from build123d import *

# Parameters (mm, degrees)
EXTRUDE_1_DEPTH = 5


with BuildPart() as part:
    # 草图1 → 凸台-拉伸1 (new body)
    with BuildSketch(Plane(origin=(0, 0, 0), x_dir=(0, 0, -1), z_dir=(1, 0, 0))):
        Polygon((0, 0), (-250, 0), (-250, 20), (-245, 20), (-245, 50), (-250, 50), (-250, 70), (0, 70), (0, 50), (-5, 50), (-5, 20), (0, 20), align=None)
        with BuildLine():
            Line((-228.2219096, 66), (-20.2219096, 66))
            ThreePointArc((-20.2219096, 66), (-19.514802819, 65.707106781), (-19.2219096, 65))
            Line((-19.2219096, 65), (-19.2219096, 64))
            ThreePointArc((-19.2219096, 64), (-19.514802819, 63.292893219), (-20.2219096, 63))
            Line((-20.2219096, 63), (-228.2219096, 63))
            ThreePointArc((-228.2219096, 63), (-228.929016382, 63.292893219), (-229.2219096, 64))
            Line((-229.2219096, 64), (-229.2219096, 65))
            ThreePointArc((-229.2219096, 65), (-228.929016382, 65.707106781), (-228.2219096, 66))
        make_face(mode=Mode.SUBTRACT)
        with BuildLine():
            Line((-228.2219096, 4), (-20.2219096, 4))
            ThreePointArc((-20.2219096, 4), (-19.514802819, 4.292893219), (-19.2219096, 5))
            Line((-19.2219096, 5), (-19.2219096, 6))
            ThreePointArc((-19.2219096, 6), (-19.514802819, 6.707106781), (-20.2219096, 7))
            Line((-20.2219096, 7), (-228.2219096, 7))
            ThreePointArc((-228.2219096, 7), (-228.929016382, 6.707106781), (-229.2219096, 6))
            Line((-229.2219096, 6), (-229.2219096, 5))
            ThreePointArc((-229.2219096, 5), (-228.929016382, 4.292893219), (-228.2219096, 4))
        make_face(mode=Mode.SUBTRACT)
    extrude(amount=EXTRUDE_1_DEPTH)


solid = part.part
The model under review builds one solid part; all positions refer to its coordinate system, in mm. A direction names the side the tool comes from. Coordinates: 2 decimals unless noted, no trailing zeros. Loops run counter-clockwise (first coordinate to the right, second up) from the corner with the lowest first, then second, coordinate; pieces in that order, holes last. Notation, with made-up numbers: M 59.25,-37 L 118.25,-37 A15 ccw 118.25,-19 Z; hole C -4.75,-30 d10. An arc over 180 degrees is marked long. Put each result on its own line as item: value. Start each with the question number.
Q1. Clearance check with flat-ended pins moving along their axes: pin 1 (2.5 mm diameter, centred on x = 2.5, z = 144.5, fed in from -Y); pin 2 (2.5 mm diameter, centred on x = 3.5, y = 40, fed in from -Z). State where each tip first meets the part, or that it passes through.
Q2. Add section A-A (z = 127.5). Write out the cut boundary in (x, y), and give its area (3 significant figures).
Q3. For faces 1 (the flat face through (2, 4, 126)), 2 (the flat face through (2, 10, 0)), 3 (the flat face through (2, 50, 2)), 4 (the flat face through (2, 35, 245)), list the 3-axis set-ups (+Z, -Z, +X, -X, +Y, -Y) from which the entire face can be reached by the end or side of a thin tool; tool diameter is ignored.
Q4. The part is to be moulded in two halves that separate along Y. For faces 5 (the flat face through (2, 70, 127)), 6 (the flat face through (2, 60, 0)), 7 (the flat face through (2, 20, 248)), say which applies: +Y half, -Y half, draft (parallel to the pull), parting line (faces both ways), or undercut.
Q5. Wall thickness on line 1 (Y direction, x = 4.5, z = 171); line 2 (Z direction, x = 1.4, y = 64); line 3 (Z direction, x = 3.55, y = 27.5): over which ranges is each line inside the solid? List them lowest first.
Q6. Add section B-B (x = 3.7). Write out the cut boundary in (y, z), and give its area (3 significant figures).
Q7. Add section C-C (y = 41.5). Write out the cut boundary in (x, z).
Answers:
1. pin 1: stops at y = 0
1. pin 2: stops at z = 5
2. outline: M 0,0 L 5,0 L 5,4 L 0,4 Z; M 0,7 L 5,7 L 5,63 L 0,63 Z; M 0,66 L 5,66 L 5,70 L 0,70 Z
2. area: 320 mm^2
3. face 1: +X, -X
3. face 2: -Z, +X, -X, +Y, -Y
3. face 3: -Z, +X, -X
3. face 4: +Z, +X, -X
4. face 5: +Y half
4. face 6: draft
4. face 7: undercut
5. line 1: y = 0 to 4, 7 to 63, 66 to 70
5. line 2: z = 0 to 19.22, 229.22 to 250
5. line 3: z = 5 to 245
6. outline: M 0,0 L 20,0 L 20,5 L 50,5 L 50,0 L 70,0 L 70,250 L 50,250 L 50,245 L 20,245 L 20,250 L 0,250 Z; hole M 4,20.22 A1 ccw 5,19.22 L 6,19.22 A1 ccw 7,20.22 L 7,228.22 A1 ccw 6,229.22 L 5,229.22 A1 ccw 4,228.22 Z; hole M 63,20.22 A1 ccw 64,19.22 L 65,19.22 A1 ccw 66,20.22 L 66,228.22 A1 ccw 65,229.22 L 64,229.22 A1 ccw 63,228.22 Z
6. area: 15,900 mm^2
7. outline: M 0,5 L 5,5 L 5,245 L 0,245 Z
